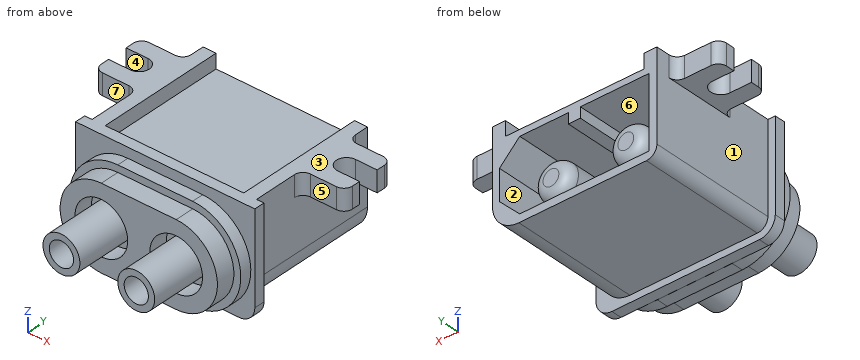
```python
from build123d import *

# Parameters (mm, degrees)
BOSS_EXTRUDE1_DEPTH        = 13.2
CUT_EXTRUDE1_DEPTH         = 8.6
BOSS_EXTRUDE2_DEPTH        = 7.1
BOSS_EXTRUDE2_DEPTH_BACK   = 11.9
SKETCH3_R                  = 1.75
BOSS_EXTRUDE2_2_DEPTH      = 7.1
BOSS_EXTRUDE2_2_DEPTH_BACK = 11.9
SKETCH4_W                  = 13.14
SKETCH4_H                  = 1.37
CUT_EXTRUDE2_DEPTH         = 12.18
BOSS_EXTRUDE3_DEPTH        = 1
BOSS_EXTRUDE4_DEPTH        = 1.1
SKETCH7_R                  = 2.5
BOSS_EXTRUDE5_DEPTH        = 1.81
SKETCH8_R                  = 1.15
CUT_EXTRUDE3_DEPTH         = 7
BOSS_EXTRUDE6_DEPTH        = 2
FILLET1_R                  = 1


with BuildPart() as part:
    # Sketch1 → Boss-Extrude1 (new body)
    with BuildSketch(Plane(origin=(0, 0, 0), x_dir=(1, 0, 0), z_dir=(0, 1, 0))):
        with BuildLine():
            Line((8.864150943, 1.753207547), (8.864150943, -5.196792453))
            Line((8.864150943, -5.196792453), (-6.735849057, -5.196792453))
            Line((-6.735849057, -5.196792453), (-6.735849057, 3.253207547))
            ThreePointArc((-6.735849057, 3.253207547), (-6.442955838, 3.960314328), (-5.735849057, 4.253207547))
            Line((-5.735849057, 4.253207547), (6.364150943, 4.253207547))
            ThreePointArc((6.364150943, 4.253207547), (8.131917896, 3.5209745), (8.864150943, 1.753207547))
        make_face()
    extrude(amount=BOSS_EXTRUDE1_DEPTH)

    # Sketch2 → Cut-Extrude1 (cut)
    with BuildSketch(Plane(origin=(0, 13.2, 0), x_dir=(1, 0, 0), z_dir=(0, 1, 0))):
        Polygon((-5.995849057, 3.523207547), (-5.995849057, -3.226792453), (0.524150943, -3.226792453), (0.524150943, -2.236792453), (1.664150943, -2.236792453), (1.664150943, -3.226792453), (6.279150943, -3.226792453), (8.204150943, -1.301792453), (8.204150943, 1.598207547), (6.279150943, 3.523207547), align=None)
    extrude(amount=-CUT_EXTRUDE1_DEPTH, mode=Mode.SUBTRACT)

    # Sketch4 → Cut-Extrude2 (cut)
    with BuildSketch(Plane(origin=(0, 13.2, 0), x_dir=(1, 0, 0), z_dir=(0, 1, 0))):
        with Locations((1.064150943, -4.511792453)):
            Rectangle(SKETCH4_W, SKETCH4_H)
    extrude(amount=-CUT_EXTRUDE2_DEPTH, mode=Mode.SUBTRACT)



with BuildPart() as body_2:
    # Sketch3 → Boss-Extrude2 (new, two sides: drawn at the far end of the back side and taken through both)
    with BuildSketch(Plane(origin=(0, 4.6, 0), x_dir=(1, 0, 0), z_dir=(0, 1, 0)).offset(-BOSS_EXTRUDE2_DEPTH_BACK)):
        with Locations(Location((-2.485849057, 0.343207547, 0), (0, 0, 270))):
            Circle(SKETCH3_R)
    extrude(amount=BOSS_EXTRUDE2_DEPTH + BOSS_EXTRUDE2_DEPTH_BACK)


with BuildPart() as body_3:
    # Sketch3 → Boss-Extrude2 2 (new, two sides: drawn at the far end of the back side and taken through both)
    with BuildSketch(Plane(origin=(0, 4.6, 0), x_dir=(1, 0, 0), z_dir=(0, 1, 0)).offset(-BOSS_EXTRUDE2_2_DEPTH_BACK)):
        with Locations(Location((4.614150943, 0.343207547, 0), (0, 0, 270))):
            Circle(SKETCH3_R)
    extrude(amount=BOSS_EXTRUDE2_2_DEPTH + BOSS_EXTRUDE2_2_DEPTH_BACK)


with BuildPart() as part_1:
    add(part.part)

    add(body_2.part)  # Boss-Extrude3 merges body 2

    add(body_3.part)  # Boss-Extrude3 merges body 3
    # Sketch5 → Boss-Extrude3 (add)
    with BuildSketch(Plane.XZ):
        with BuildLine():
            Line((-7.435849057, 5.196792453), (9.564150943, 5.196792453))
            Line((9.564150943, 5.196792453), (9.564150943, -3.403207547))
            ThreePointArc((9.564150943, -3.403207547), (9.124811115, -4.463867719), (8.064150943, -4.903207547))
            Line((8.064150943, -4.903207547), (-5.935849057, -4.903207547))
            ThreePointArc((-5.935849057, -4.903207547), (-6.996509228, -4.463867719), (-7.435849057, -3.403207547))
            Line((-7.435849057, -3.403207547), (-7.435849057, 5.196792453))
        make_face()
    extrude(amount=-BOSS_EXTRUDE3_DEPTH)

    # Sketch6 → Boss-Extrude4 (add)
    with BuildSketch(Plane.XZ):
        with BuildLine():
            Line((-2.485849057, 4.226792453), (4.614150943, 4.226792453))
            ThreePointArc((4.614150943, 4.226792453), (9.184150943, -0.343207547), (4.614150943, -4.913207547))
            Line((4.614150943, -4.913207547), (-2.485849057, -4.913207547))
            ThreePointArc((-2.485849057, -4.913207547), (-7.055849057, -0.343207547), (-2.485849057, 4.226792453))
        make_face()
    extrude(amount=BOSS_EXTRUDE4_DEPTH)

    # Sketch7 → Boss-Extrude5 (add)
    with BuildSketch(Plane(origin=(0, -1.1, 0), x_dir=(-1, 0, 0), z_dir=(0, -1, 0))):
        with BuildLine():
            Line((2.485849057, -3.566792453), (-4.614150943, -3.566792453))
            ThreePointArc((-4.614150943, -3.566792453), (-8.524150943, 0.343207547), (-4.614150943, 4.253207547))
            Line((-4.614150943, 4.253207547), (2.485849057, 4.253207547))
            ThreePointArc((2.485849057, 4.253207547), (6.395849057, 0.343207547), (2.485849057, -3.566792453))
        make_face()
        with Locations(Location((2.485849057, 0.343207547, 0), (0, 0, 270))):
            Circle(SKETCH7_R, mode=Mode.SUBTRACT)
        with Locations(Location((-4.614150943, 0.343207547, 0), (0, 0, 270))):
            Circle(SKETCH7_R, mode=Mode.SUBTRACT)
    extrude(amount=BOSS_EXTRUDE5_DEPTH)

    # Sketch8 → Cut-Extrude3 (cut)
    with BuildSketch(Plane.XZ.offset(7.3)):
        with Locations(Location((4.614150943, -0.343207547, 0), (0, 0, 270))):
            Circle(SKETCH8_R)
        with Locations(Location((-2.485849057, -0.343207547, 0), (0, 0, 270))):
            Circle(SKETCH8_R)
    extrude(amount=-CUT_EXTRUDE3_DEPTH, mode=Mode.SUBTRACT)

    # Sketch9 → Boss-Extrude6 (add)
    with BuildSketch(Plane.XY.offset(5.196792453)):
        with BuildLine():
            Line((-7.535849057, 11.09), (-10.042204833, 11.09))
            ThreePointArc((-10.042204833, 11.09), (-10.607890258, 10.855685425), (-10.842204833, 10.29))
            Line((-10.842204833, 10.29), (-10.842204833, 9.50439657))
            Line((-10.842204833, 9.50439657), (-8.785849057, 9.50439657))
            ThreePointArc((-8.785849057, 9.50439657), (-7.816452486, 8.535), (-8.785849057, 7.56560343))
            Line((-8.785849057, 7.56560343), (-10.842204833, 7.56560343))
            Line((-10.842204833, 7.56560343), (-10.842204833, 6.78))
            ThreePointArc((-10.842204833, 6.78), (-10.607890258, 6.214314575), (-10.042204833, 5.98))
            Line((-10.042204833, 5.98), (-7.535849057, 5.98))
            ThreePointArc((-7.535849057, 5.98), (-6.970163632, 5.745685425), (-6.735849057, 5.18))
            Line((-6.735849057, 5.18), (-6.735849057, 11.89))
            ThreePointArc((-6.735849057, 11.89), (-6.970163632, 11.324314575), (-7.535849057, 11.09))
        make_face()
        with BuildLine():
            Line((12.97050672, 7.56560343), (12.97050672, 6.78))
            ThreePointArc((12.97050672, 6.78), (12.736192145, 6.214314575), (12.17050672, 5.98))
            Line((12.17050672, 5.98), (9.664150943, 5.98))
            ThreePointArc((9.664150943, 5.98), (9.098465518, 5.745685425), (8.864150943, 5.18))
            Line((8.864150943, 5.18), (8.864150943, 11.89))
            ThreePointArc((8.864150943, 11.89), (9.098465518, 11.324314575), (9.664150943, 11.09))
            Line((9.664150943, 11.09), (12.17050672, 11.09))
            ThreePointArc((12.17050672, 11.09), (12.736192145, 10.855685425), (12.97050672, 10.29))
            Line((12.97050672, 10.29), (12.97050672, 9.50439657))
            Line((12.97050672, 9.50439657), (10.914150943, 9.50439657))
            ThreePointArc((10.914150943, 9.50439657), (9.944754373, 8.535), (10.914150943, 7.56560343))
            Line((10.914150943, 7.56560343), (12.97050672, 7.56560343))
        make_face()
    extrude(amount=-BOSS_EXTRUDE6_DEPTH)

    # Fillet1
    fillet1_edges = [part_1.edges().sort_by_distance(p)[0] for p in [
        (-2.485849057, 11.7, -2.093207547),
        (4.614150943, 11.7, -2.093207547),
    ]]
    fillet(fillet1_edges, radius=FILLET1_R)


solid = part_1.part
```
For this review, take the finished solid that the model builds, in its own axes (mm). Face numbers are marked on the shaded views. A direction names the side the tool comes from. Give positions to 0.01 mm unless a question says otherwise; leave off trailing zeros. Write each loop counter-clockwise with the first axis right and the second up, starting at its lowest first coordinate (ties: lowest second). Pieces come first, ordered by that corner, then holes. Notation, with made-up numbers: M -18,87.5 L 17,87.5 A18 cw 17,99.5 Z; hole C 12,40 d5. An arc over 180 degrees is marked long. Answer as CSV lines item,"result".
1. For the marked faces 4, 5, 6 and 7, list the 3-axis set-ups (+Z, -Z, +X, -X, +Y, -Y) from which the entire face can be reached by the end or side of a thin tool; tool diameter is ignored.
Findings:
face 4,"+Z, -Z, -X"
face 5,"+Z, -Z, +X, -Y"
face 6,"+Y"
face 7,"+Z, -Z, -X, -Y"
2. Consider section B-B, the plane x = -9.25. Write out the cut boundary in (y, z).
Findings:
outline,"M 5.98,3.2 L 7.57,3.2 L 7.57,5.2 L 5.98,5.2 Z; M 9.5,3.2 L 11.09,3.2 L 11.09,5.2 L 9.5,5.2 Z"
3. Consider section D-D, the plane y = -5.25. Write out the cut boundary in (x, z), then the cut area to 3 significant figures.
Findings:
outline,"C -2.49,-0.34 d3.5; C 4.61,-0.34 d3.5; hole C -2.49,-0.34 d2.3; hole C 4.61,-0.34 d2.3"
area,"10.9 mm2"
4. Consider section A-A, the plane y = -1.75. Write out the cut boundary in (x, z).
Findings:
outline,"C -2.49,-0.34 d3.5; M -2.49,-4.25 L 4.61,-4.25 A3.91 ccw 4.61,3.57 L -2.49,3.57 A3.91 ccw Z; C 4.61,-0.34 d3.5; hole C -2.49,-0.34 d5; hole C -2.49,-0.34 d2.3; hole C 4.61,-0.34 d5; hole C 4.61,-0.34 d2.3"
5. For pin 1 (3.5 mm diameter, centred on x = -1, z = -0.5, fed in from +Y); pin 2 (0.7 mm diameter, centred on x = 0, z = 4.5, fed in from +Y); pin 3 (2 mm diameter, centred on y = -4.5, z = 0.5, fed in from +X); pin 4 (3 mm diameter, centred on x = 5, z = -3.5, fed in from +Y), all flat-tipped, find the tip position at first contact; note any pin that passes through.
Findings:
pin 1,"stops at y = 11.7"
pin 2,"stops at y = 1.02"
pin 3,"stops at x = 6.36"
pin 4,"stops at y = 13.2"
6. Wall thickness on line 1 (X direction, y = 11, z = -1.5); line 2 (X direction, y = 5.5, z = 1.25); line 3 (Z direction, x = 4, y = 11.5): over which ranges is each line inside the solid? List them lowest first.
Findings:
line 1,"x = -6.74 to -6, -3.74 to -1.23, 3.36 to 5.87, 8.2 to 8.86"
line 2,"x = -6.74 to -6, -3.21 to -1.76, 3.89 to 5.34, 8.2 to 8.86"
line 3,"z = -4.25 to -3.52, -1.55 to 0.86, 3.23 to 3.83"
7. Consider section C-C, the plane y = 8.75. Write out the cut boundary in (x, z), then the cut area to 3 significant figures.
Findings:
outline,"M -7.84,3.2 L -6.74,3.2 L -6.74,-3.25 A1 ccw -5.74,-4.25 L 6.36,-4.25 A2.5 ccw 8.86,-1.75 L 8.86,3.2 L 9.97,3.2 L 9.97,5.2 L 7.63,5.2 L 7.63,3.83 L -5.51,3.83 L -5.51,5.2 L -7.84,5.2 Z; C -2.49,-0.34 d3.5; C 4.61,-0.34 d3.5; hole M -6,-3.52 L 6.28,-3.52 L 8.2,-1.6 L 8.2,1.3 L 6.28,3.23 L 1.66,3.23 L 1.66,2.24 L 0.52,2.24 L 0.52,3.23 L -6,3.23 Z"
area,"60.5 mm2"
8. Draft analysis for pull direction X (two halves, no side actions). For the marked faces 1, 2 and 3, state which applies: +X half, -X half, draft (parallel to the pull), parting line (faces both ways), or undercut.
Findings:
face 1,"-X half"
face 2,"undercut"
face 3,"draft"
